```python
from build123d import *

# Parameters (mm, degrees)
F0_R     = 1
F0_W     = 7.5
F0_H     = 5.5
F0_W_2   = 8
F0_H_2   = 7.5
F0_R_2   = 2.75
F0_H_3   = 0.5
F1_DEPTH = 1
F2_DEPTH = 3.5
F3_DEPTH = 5
F4_DEPTH = 6
F5_DEPTH = 2.5


with BuildPart() as f1:
    # F0 (on Top) → F1 (new body, symmetric)
    with BuildSketch(Plane.XY):
        Polygon((-10.037144646, -6), (-10.037144646, -12), (10.962855354, -12), (10.962855354, -6), (4, -6), (4, -6.5), (-4, -6.5), (-4, -6), align=None)
        Polygon((12.5, 12), (-12.5, 12), (-12.5, -12), (-10.037144646, -12), (-10.037144646, -6), (-4, -6), (-4, 1.5), (4, 1.5), (4, -6), (10.962855354, -6), (10.962855354, -12), (12.5, -12), align=None)
        with Locations((-10.5, -2.5)):
            Circle(F0_R, mode=Mode.SUBTRACT)
        with Locations((10.5, -2.5)):
            Circle(F0_R, mode=Mode.SUBTRACT)
        with Locations((-10.5, 10)):
            Circle(F0_R, mode=Mode.SUBTRACT)
        with Locations((0, 7.75)):
            Rectangle(F0_W, F0_H, mode=Mode.SUBTRACT)
        with Locations((10.5, 10)):
            Circle(F0_R, mode=Mode.SUBTRACT)
        with Locations((0, 7.75)):
            Rectangle(F0_W, F0_H)
        with Locations((0, -2.25)):
            Rectangle(F0_W_2, F0_H_2)
        with Locations((0, -2.5)):
            Circle(F0_R_2, mode=Mode.SUBTRACT)
        with Locations((0, -2.5)):
            Circle(F0_R_2)
        with Locations((0, -6.25)):
            Rectangle(F0_W_2, F0_H_3)
    extrude(amount=F1_DEPTH, both=True)

    # F0 (on Top) → F2 (join)
    with BuildSketch(Plane.XY):
        Polygon((-10.037144646, -6), (-10.037144646, -12), (10.962855354, -12), (10.962855354, -6), (4, -6), (4, -6.5), (-4, -6.5), (-4, -6), align=None)
        with Locations((0, -6.25)):
            Rectangle(F0_W_2, F0_H_3)
    extrude(amount=-F2_DEPTH)

    # F0 (on Top) → F3 (join)
    with BuildSketch(Plane.XY):
        with Locations((0, -2.25)):
            Rectangle(F0_W_2, F0_H_2)
        with Locations((0, -2.5)):
            Circle(F0_R_2, mode=Mode.SUBTRACT)
        with Locations((0, -2.5)):
            Circle(F0_R_2)
        with Locations((0, -6.25)):
            Rectangle(F0_W_2, F0_H_3)
    extrude(amount=F3_DEPTH)

    # F0 (on Top) → F4 (join)
    with BuildSketch(Plane.XY):
        with Locations((0, -2.5)):
            Circle(F0_R_2)
    extrude(amount=F4_DEPTH)

    # F0 (on Top) → F5 (join)
    with BuildSketch(Plane.XY):
        with Locations((0, 7.75)):
            Rectangle(F0_W, F0_H)
    extrude(amount=F5_DEPTH)


solid = f1.part
```
Model file for the job. Use its own axes, mm. A direction names the side the tool comes from. Give positions to 0.01 mm unless a question says otherwise; leave off trailing zeros. Loops run counter-clockwise (first coordinate to the right, second up) from the corner with the lowest first, then second, coordinate; pieces in that order, holes last. Notation, with made-up numbers: M 46.25,-14.75 L 95.25,-14.75 A5 ccw 95.25,-8.75 Z; hole C -5,58 d7. An arc over 180 degrees is marked long. Use one line per item in the form item = value.
Item 1: Slice it at D-D on x = 3.25. List the corners of the cut face in (y, z), and give its area (3 significant figures).
Filled in:
outline = M -12,-3.5 L -6,-3.5 L -6,-1 L 12,-1 L 12,1 L 10.5,1 L 10.5,2.5 L 5,2.5 L 5,1 L 1.5,1 L 1.5,5 L -6.5,5 L -6.5,1 L -12,1 Z
area = 103 mm^2
Item 2: Slice it at A-A on z = 2. List the corners of the cut face in (x, y), and give its area (3 significant figures).
Filled in:
outline = M -4,-6.5 L 4,-6.5 L 4,1.5 L -4,1.5 Z; M -3.75,5 L 3.75,5 L 3.75,10.5 L -3.75,10.5 Z
area = 105 mm^2
Item 3: Flat gauge pins, fed straight in: pin 1 Ø3 at (y, z) = (-5.5, 3.5) entering from +X; pin 2 Ø3 at (x, y) = (-2, 7) entering from +Z; pin 3 Ø2 at (y, z) = (-10, -3) entering from -X; pin 4 Ø3 at (x, z) = (4.5, -1.5) entering from +Y. Where does each tip first touch, or does it go through?
Filled in:
pin_1 = 4
pin_2 = 2.5
pin_3 = -10.04
pin_4 = 12
Item 4: Two-plate mould, pull along X, no slides. Class faces 6 (the flat face through (0, -6.5, 3)), 7 (the flat face through (3.75, 8, 2)), 8 (the flat face through (-12.5, 0, 0)), 9 (the cylindrical face through (10.37, 10.99, -0.01)): released by +X, released by -X, zero draft, split by the parting line, or undercut.
Filled in:
face_6 = zero draft
face_7 = released by +X
face_8 = released by -X
face_9 = undercut
Item 5: Slice it at C-C on x = 10.5. List the corners of the cut face in (y, z), and give its area (3 significant figures).
Filled in:
outline = M -12,-3.5 L -6,-3.5 L -6,-1 L -3.5,-1 L -3.5,1 L -12,1 Z; M -1.5,-1 L 9,-1 L 9,1 L -1.5,1 Z; M 11,-1 L 12,-1 L 12,1 L 11,1 Z
area = 55.0 mm^2
Item 6: Drill centre lines: L1, parallel to Y at x = -10.5, z = 0.45; L2, parallel to Z at x = 2.25, y = 0.5; L3, parallel to X at y = 7, z = 1.25. Where is each one in solid material? Low to high.
Filled in:
L1 = -12 to -3.5, -1.5 to 9, 11 to 12
L2 = -1 to 5
L3 = -3.75 to 3.75
Item 7: Slice it at B-B on y = -2.5. List the corners of the cut face in (x, z).
Filled in:
outline = M -12.5,-1 L -11.5,-1 L -11.5,1 L -12.5,1 Z; M -9.5,-1 L 9.5,-1 L 9.5,1 L 4,1 L 4,5 L 2.75,5 L 2.75,6 L -2.75,6 L -2.75,5 L -4,5 L -4,1 L -9.5,1 Z; M 11.5,-1 L 12.5,-1 L 12.5,1 L 11.5,1 Z
Item 8: Which spindle directions (+Z, -Z, +X, -X, +Y, -Y) get a long thin tool onto all of the face, cutting with end or side? Do faces 1 (the flat face through (10.963, -9, -2)), 2 (the flat face through (0, 1.5, 3)), 3 (the flat face through (-10.037, -9, -2)), 4 (the flat face through (1, -6, -2)), 5 (the flat face through (0, 10.5, 2)). Say none if no direction does.
Filled in:
face_1 = -Z, +X, +Y, -Y
face_2 = +Z, +X, -X
face_3 = -Z, -X, +Y, -Y
face_4 = -Z, +X, -X, +Y
face_5 = +Z, +X, -X, +Y
